CAD build for the part. Positions are in the model's coordinates, mm. Face numbers are marked on the shaded views. Coordinates: 2 decimals unless noted, no trailing zeros. Order: outer loops, then holes, each group sorted by start corner. A loop starts at its lowest first (then second) coordinate and runs counter-clockwise, first axis right, second up. Notation, with made-up numbers: (52, 81) -> (81, 81) arc R31 ccw to (81, 111) -> close; hole circle Ø6 at (19.25, 43.25). An arc over 180 degrees is marked (long way). Use one line per item in the form item = value. Start each with the question number.
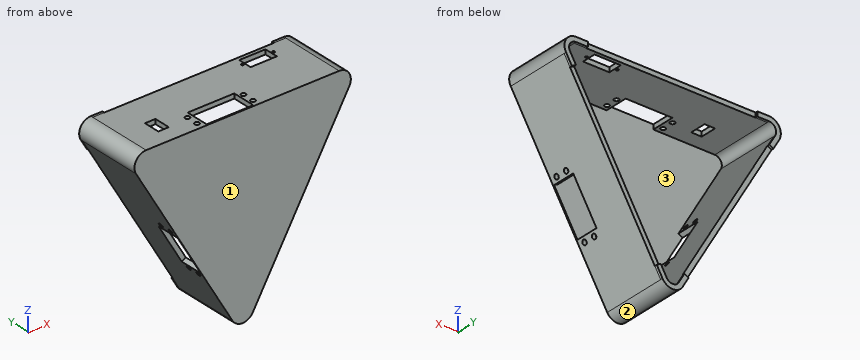
from build123d import *

# Parameters (mm, degrees)
BOSS_EXTRUDE1_DEPTH = 1
BOSS_EXTRUDE2_DEPTH = 55
BOSS_EXTRUDE3_START = -56
BOSS_EXTRUDE3_DEPTH = 58
SKETCH3_R           = 2
SKETCH3_R_2         = 1
SKETCH3_W           = 40
SKETCH3_H           = 20
SKETCH3_W_2         = 22.5
SKETCH3_H_2         = 12
SKETCH3_W_3         = 9
SKETCH3_H_3         = 14
BACK_DEPTH          = 10
SKETCH6_R           = 2
SKETCH6_W           = 40
SKETCH6_H           = 20
CUT_EXTRUDE3_DEPTH  = 10
SKETCH7_R           = 2
SKETCH7_W           = 40
SKETCH7_H           = 20
CUT_EXTRUDE4_DEPTH  = 10
CIRPATTERN1_COUNT   = 3


with BuildPart() as part:
    # Sketch2 → Boss-Extrude1 (new body)
    with BuildSketch(Plane(origin=(0, 0, 0), x_dir=(1, 0, 0), z_dir=(0, 1, 0))):
        with BuildLine():
            Line((-8.660254038, 100.470053838), (-91.339745962, -42.735026919))
            ThreePointArc((-91.339745962, -42.735026919), (-91.339745962, -52.735026919), (-82.679491924, -57.735026919))
            Line((-82.679491924, -57.735026919), (82.679491924, -57.735026919))
            ThreePointArc((82.679491924, -57.735026919), (91.339745962, -52.735026919), (91.339745962, -42.735026919))
            Line((91.339745962, -42.735026919), (8.660254038, 100.470053838))
            ThreePointArc((8.660254038, 100.470053838), (0, 105.470053838), (-8.660254038, 100.470053838))
        make_face()
    extrude(amount=-BOSS_EXTRUDE1_DEPTH)

    # Sketch2<6> → Boss-Extrude2 (add)
    with BuildSketch(Plane(origin=(0, 0, 0), x_dir=(1, 0, 0), z_dir=(0, 1, 0))):
        with BuildLine():
            Line((-8.660254038, 100.470053838), (-91.339745962, -42.735026919))
            ThreePointArc((-91.339745962, -42.735026919), (-91.339745962, -52.735026919), (-82.679491924, -57.735026919))
            Line((-82.679491924, -57.735026919), (82.679491924, -57.735026919))
            ThreePointArc((82.679491924, -57.735026919), (91.339745962, -52.735026919), (91.339745962, -42.735026919))
            Line((91.339745962, -42.735026919), (8.660254038, 100.470053838))
            ThreePointArc((8.660254038, 100.470053838), (0, 105.470053838), (-8.660254038, 100.470053838))
        make_face()
        with BuildLine():
            Line((-5.196152423, 98.470053838), (-87.875644347, -44.735026919))
            ThreePointArc((-87.875644347, -44.735026919), (-87.875644347, -50.735026919), (-82.679491924, -53.735026919))
            Line((-82.679491924, -53.735026919), (82.679491924, -53.735026919))
            ThreePointArc((82.679491924, -53.735026919), (87.875644347, -50.735026919), (87.875644347, -44.735026919))
            Line((87.875644347, -44.735026919), (5.196152423, 98.470053838))
            ThreePointArc((5.196152423, 98.470053838), (0, 101.470053838), (-5.196152423, 98.470053838))
        make_face(mode=Mode.SUBTRACT)
    extrude(amount=BOSS_EXTRUDE2_DEPTH)

    # Sketch4 → Boss-Extrude3 (add)
    with BuildSketch(Plane(origin=(0, 55, 0), x_dir=(1, 0, 0), z_dir=(0, 1, 0)).offset(BOSS_EXTRUDE3_START)):
        with BuildLine():
            Line((0, 105.470053838), (0, 101.470053838))
            ThreePointArc((0, 101.470053838), (-3, 100.666206261), (-5.196152423, 98.470053838))
            Line((-5.196152423, 98.470053838), (-10.196152423, 89.8097998))
            Line((-10.196152423, 89.8097998), (-13.660254038, 91.8097998))
            Line((-13.660254038, 91.8097998), (-8.660254038, 100.470053838))
            ThreePointArc((-8.660254038, 100.470053838), (-5, 104.130307876), (0, 105.470053838))
        make_face()
        with BuildLine():
            Line((-82.875644347, -36.074772881), (-86.339745962, -34.074772881))
            Line((-86.339745962, -34.074772881), (-91.339745962, -42.735026919))
            ThreePointArc((-91.339745962, -42.735026919), (-92.679491924, -47.735026919), (-91.339745962, -52.735026919))
            Line((-91.339745962, -52.735026919), (-87.875644347, -50.735026919))
            ThreePointArc((-87.875644347, -50.735026919), (-88.679491924, -47.735026919), (-87.875644347, -44.735026919))
            Line((-87.875644347, -44.735026919), (-82.875644347, -36.074772881))
        make_face()
    boss_extrude3 = extrude(amount=BOSS_EXTRUDE3_DEPTH)

    # Sketch3 → Back (cut)
    with BuildSketch(Plane.XY.offset(57.735026919)):
        with Locations((-34.24280037, 15)):
            Circle(SKETCH3_R)
        with Locations((-34.24280037, 5)):
            Circle(SKETCH3_R)
        with Locations((13.75719963, 15)):
            Circle(SKETCH3_R)
        with Locations((13.75719963, 5)):
            Circle(SKETCH3_R)
        with Locations((38.339745962, 46)):
            Circle(SKETCH3_R_2)
        with Locations((64.839745962, 46)):
            Circle(SKETCH3_R_2)
        with Locations((-10, 10)):
            Rectangle(SKETCH3_W, SKETCH3_H)
        with Locations((51.589745962, 46)):
            Rectangle(SKETCH3_W_2, SKETCH3_H_2)
        with Locations((-56.339745962, 20)):
            Rectangle(SKETCH3_W_3, SKETCH3_H_3)
    extrude(amount=-BACK_DEPTH, mode=Mode.SUBTRACT)

    # Sketch6 → Cut-Extrude3 (cut)
    with BuildSketch(Plane(origin=(50, 0, -28.867513459), x_dir=(-0.5, 0, -0.866025404), z_dir=(0.866025404, 0, -0.5))):
        with Locations((-14, 15)):
            Circle(SKETCH6_R)
        with Locations((-14, 5)):
            Circle(SKETCH6_R)
        with Locations((34, 15)):
            Circle(SKETCH6_R)
        with Locations((34, 5)):
            Circle(SKETCH6_R)
        with Locations((10, 10)):
            Rectangle(SKETCH6_W, SKETCH6_H)
    extrude(amount=-CUT_EXTRUDE3_DEPTH, mode=Mode.SUBTRACT)

    # Sketch7 → Cut-Extrude4 (cut)
    with BuildSketch(Plane(origin=(-50, 0, -28.867513459), x_dir=(-0.5, 0, 0.866025404), z_dir=(-0.866025404, 0, -0.5))):
        with Locations((-34, 15)):
            Circle(SKETCH7_R)
        with Locations((-34, 5)):
            Circle(SKETCH7_R)
        with Locations((14, 15)):
            Circle(SKETCH7_R)
        with Locations((14, 5)):
            Circle(SKETCH7_R)
        with Locations((-10, 10)):
            Rectangle(SKETCH7_W, SKETCH7_H)
    extrude(amount=-CUT_EXTRUDE4_DEPTH, mode=Mode.SUBTRACT)

    # CirPattern1: Boss-Extrude3 ×3 about axis
    cirpattern1_axis = Axis((0, 0, 0), (0, 1, 0))
    for i in range(1, CIRPATTERN1_COUNT):
        add(boss_extrude3.rotate(cirpattern1_axis, i * 360 / CIRPATTERN1_COUNT))


solid = part.part
1) Two-plate mould, pull along X, no slides. Class the marked faces 1, 2 and 3: released by +X, released by -X, zero draft, split by the parting line, or undercut.
2) Drop flat-ended pins along their axis: P1, Ø4.5, axis at y = 46, z = 56.5, coming from the +X side; P2, Ø4.5, axis at y = 23, z = 56.5, coming from the -X side; P3, Ø3.5, axis at x = 13.76, y = 5, coming from the +Z side. Give the stop position or say it passes through.
3) Cut at B-B on x = -39.5. Give the cut face in (y, z), then the cut area to 3 significant figures.
4) Probe L1, parallel to Z at x = -41, y = 16; L2, parallel to Z at x = -35.5, y = 45; L3, parallel to X at y = 54.5, z = 9.5. List the from-to ranges inside material, lowest first.
5) Cut at C-C on x = -75.5. Give the cut face in (y, z), then the cut area to 3 significant figures.
6) Cut at D-D on z = 0.5. Give the cut face in (x, y), then the cut area to 3 significant figures.
7) Cut at A-A on y = 37. Give the cut face in (x, z), then the cut area to 3 significant figures.
Values follow:
q1.face_1 = zero draft
q1.face_2 = split by the parting line
q1.face_3 = undercut
q2.P1 = 90.27
q2.P2 = -90.27
q2.P3 = -80.61
q3.outline = (-1, -47.05) -> (0, -47.05) -> (0, 53.74) -> (55, 53.74) -> (55, 57.74) -> (-1, 57.74) -> close; (20, -47.05) -> (55, -47.05) -> (55, -39.05) -> (20, -39.05) -> close
q3.area = 605 mm^2
q4.L1 = 53.74 to 57.74
q4.L2 = -53.98 to -45.98, 53.74 to 57.74
q4.L3 = -72.15 to -67.53, 67.53 to 72.15
q5.outline = (-1, 15.3) -> (55, 15.3) -> (55, 23.3) -> (0, 23.3) -> (0, 53.74) -> (57, 53.74) -> (57, 57.74) -> (-1, 57.74) -> close
q5.area = 710 mm^2
q6.outline = (-66.96, -1) -> (66.96, -1) -> (66.96, 55) -> (62.34, 55) -> (62.34, 0) -> (-62.34, 0) -> (-62.34, 55) -> (-66.96, 55) -> close
q6.area = 642 mm^2
q7.outline = (-91.34, 42.74) -> (-8.66, -100.47) arc R10 ccw to (8.66, -100.47) -> (91.34, 42.74) arc R10 ccw to (82.68, 57.74) -> (-82.68, 57.74) arc R10 ccw to start; hole (-87.88, 44.74) -> (-5.2, -98.47) arc R6 ccw to (5.2, -98.47) -> (87.88, 44.74) arc R6 ccw to (82.68, 53.74) -> (-82.68, 53.74) arc R6 ccw to start
q7.area = 2,190 mm^2
